The model under review builds one solid part; all positions refer to its coordinate system, in mm. Give positions to 0.01 mm unless a question says otherwise; leave off trailing zeros. Order: outer loops, then holes, each group sorted by start corner. A loop starts at its lowest first (then second) coordinate and runs counter-clockwise, first axis right, second up. Notation, with made-up numbers: (-33, -9.5) - (10, -9.5) arc R30 ccw to (10, 23.5) - close; hole circle Ø3 at (14.5, 25). An arc over 180 degrees is marked (long way). Put each result on its own line as item: value.
```python
from build123d import *

# Parameters (mm, degrees)
ESQUISSE4_R        = 1.55
ESQUISSE4_R_2      = 4
ESQUISSE4_R_3      = 5
ESQUISSE4_R_4      = 1.35255
ESQUISSE4_R_5      = 2.7051
BOSS_EXTRU_3_DEPTH = 3


with BuildPart() as part:
    # Esquisse4 → Boss.-Extru.3 (new body)
    with BuildSketch(Plane(origin=(0, 0, 0), x_dir=(0, 0, -1), z_dir=(1, 0, 0))):
        with BuildLine():
            Line((-40.60825, -12.7), (-40.60825, -16.144875))
            Line((-40.60825, -16.144875), (-40.60825, -16.348305132))
            add(Edge.make_bspline(
                [(-40.60825, -16.348305132), (-40.365634485, -16.661193605), (-40.112338127, -16.96547542), (-39.63020507, -17.593748723), (-39.400688032, -17.917191992), (-38.719045939, -18.893089111), (-38.271947044, -19.549593057), (-37.338540998, -20.831006808), (-36.855460104, -21.458516341), (-36.059725811, -22.342477591), (-35.781944124, -22.627029047), (-35.202868212, -23.17718548), (-34.900674383, -23.443503751), (-33.971943166, -24.212706181), (-33.324405882, -24.685383849), (-32.010805282, -25.604549776), (-31.348089528, -26.055770333), (-30.303090708, -26.660610546), (-29.948270215, -26.848696892), (-29.222483721, -27.184971005), (-28.851412004, -27.333773538), (-28.083597976, -27.570691368), (-27.685315555, -27.657976057), (-27.090666934, -27.715403346), (-26.891908645, -27.722631025), (-26.592836888, -27.712936491), (-26.492990431, -27.706278992), (-26.292963936, -27.685632014), (-26.192732932, -27.670522326), (-26.092449031, -27.65425)],
                knots=[0, 0, 0, 0, 0.0625, 0.0625, 0.125, 0.125, 0.25, 0.25, 0.375, 0.375, 0.4375, 0.4375, 0.5, 0.5, 0.625, 0.625, 0.75, 0.75, 0.8125, 0.8125, 0.875, 0.875, 0.9375, 0.9375, 0.96875, 0.96875, 0.984375, 0.984375, 1, 1, 1, 1], degree=3))
            Line((-26.092449031, -27.65425), (-26.092449031, -90))
            ThreePointArc((-26.092449031, -90), (2.64551669, -116.14013034), (25.954024412, -85.06135051))
            Line((25.954024412, -85.06135051), (25.954024412, -27.65425))
            add(Edge.make_bspline(
                [(25.954024412, -27.65425), (27.179118802, -27.419536533), (28.353377808, -27.051803075), (30.05705383, -26.34918771), (30.615126485, -26.089288473), (31.712904721, -25.521429223), (32.254485024, -25.212118815), (33.827204106, -24.230350536), (34.814025463, -23.502087852), (36.672007358, -21.907218093), (37.543320305, -21.040793316), (38.751902771, -19.623473398), (39.134714509, -19.134962989), (39.851014333, -18.131439591), (40.185535135, -17.615291382), (40.801362362, -16.550595558), (41.082635497, -16.002027673), (41.457015911, -15.150237789), (41.574249194, -14.86042264), (41.789713906, -14.277065554), (41.888049248, -13.98351322), (42.334688534, -12.506770959), (42.546239761, -11.296312151), (42.717568356, -9.451511475), (42.750611649, -8.83067761), (42.772859866, -7.900507946), (42.775360474, -7.590422151), (42.77555993, -6.970221998), (42.772087252, -6.66010067), (42.772087252, -6.35)],
                knots=[0, 0, 0, 0, 0.125, 0.125, 0.1875, 0.1875, 0.25, 0.25, 0.375, 0.375, 0.5, 0.5, 0.5625, 0.5625, 0.625, 0.625, 0.6875, 0.6875, 0.71875, 0.71875, 0.75, 0.75, 0.875, 0.875, 0.9375, 0.9375, 0.96875, 0.96875, 1, 1, 1, 1], degree=3))
            add(Edge.make_bspline(
                [(42.772087252, -6.35), (42.772087252, -5.874878454), (42.783792207, -5.398095979), (42.789657917, -4.447020546), (42.781867467, -3.973004463), (42.672546396, -2.563152451), (42.499179213, -1.637510108), (42.106282017, -0.267897459), (41.954068536, 0.185625042), (41.614819435, 1.087728793), (41.430081297, 1.530283034), (40.844911495, 2.839259084), (40.416604561, 3.689518781), (39.046783283, 6.190525131), (38.013123304, 7.787251584), (36.291657446, 10.082106977), (35.688509547, 10.830664164), (34.43654182, 12.281738953), (33.786199883, 12.985690235), (33.112075, 13.668565083)],
                knots=[0, 0, 0, 0, 0.0625, 0.0625, 0.125, 0.125, 0.25, 0.25, 0.3125, 0.3125, 0.375, 0.375, 0.5, 0.5, 0.75, 0.75, 0.875, 0.875, 1, 1, 1, 1], degree=3))
            add(Edge.make_bspline(
                [(33.112075, 13.668565083), (32.332207955, 14.539101946), (31.435060987, 15.277734234)],
                knots=[0, 0, 0, 1, 1, 1], degree=2))
            add(Edge.make_bspline(
                [(31.435060987, 15.277734234), (30.299691041, 16.309376592), (29.113704516, 17.275445235), (26.646604831, 19.084346085), (25.360475951, 19.928267183), (21.432297769, 22.265681686), (18.70167828, 23.563722979), (14.477833082, 25.213127628), (13.049229105, 25.71486416), (10.864398428, 26.369911185), (10.129061703, 26.571832136), (8.64156399, 26.936524394), (7.890831572, 27.098844789), (5.637990782, 27.512412208), (4.127431428, 27.693727696), (2.225306731, 27.768676851), (1.844136038, 27.775542931), (1.080940786, 27.779973661), (0.698904769, 27.777413484), (-0.446346689, 27.779064109), (-1.208874123, 27.797823926), (-2.732682239, 27.815308111), (-3.492085471, 27.806304753), (-5.004084105, 27.739990771), (-5.756994671, 27.684916502), (-8.006157922, 27.451797552), (-9.492662784, 27.204583891), (-11.701987236, 26.688775277), (-12.434852331, 26.491461598), (-13.894254142, 26.051929085), (-14.622118919, 25.807493497), (-16.765417144, 25.01223388), (-18.151500369, 24.400517874), (-20.847821735, 23.032525232), (-22.158708475, 22.277484827), (-24.716496252, 20.645447351), (-25.966430559, 19.7652326), (-28.39125747, 17.919703458), (-29.567431908, 16.954258357), (-31.287557173, 15.454109034), (-31.85380584, 14.945666112), (-32.972832423, 13.91291508), (-33.52577931, 13.388805977), (-34.066096443, 12.849822171)],
                knots=[0, 0, 0, 0, 0.0625, 0.0625, 0.125, 0.125, 0.25, 0.25, 0.3125, 0.3125, 0.34375, 0.34375, 0.375, 0.375, 0.4375, 0.4375, 0.453125, 0.453125, 0.46875, 0.46875, 0.5, 0.5, 0.53125, 0.53125, 0.5625, 0.5625, 0.625, 0.625, 0.65625, 0.65625, 0.6875, 0.6875, 0.75, 0.75, 0.8125, 0.8125, 0.875, 0.875, 0.9375, 0.9375, 0.96875, 0.96875, 1, 1, 1, 1], degree=3))
            add(Edge.make_bspline(
                [(-34.066096443, 12.849822171), (-35.159801618, 11.692162737), (-36.251081621, 10.53740284), (-37.166580532, 9.404947171)],
                knots=[0, 0, 0, 0, 1, 1, 1, 1], degree=3))
            ThreePointArc((-37.166580532, 9.404947171), (-37.363014685, 9.160281042), (-37.557796616, 8.914297524))
            add(Edge.make_bspline(
                [(-37.557796616, 8.914297524), (-38.142933539, 8.170182683), (-38.709522845, 7.412667282), (-39.741912272, 5.824816801), (-40.203133529, 4.998794666), (-40.60825, 4.142494902)],
                knots=[0, 0, 0, 0, 0.5, 0.5, 1, 1, 1, 1], degree=3))
            Line((-40.60825, 4.142494902), (-40.60825, -12.7))
        make_face()
        with Locations((0.1651, -103.128774516)):
            Circle(ESQUISSE4_R, mode=Mode.SUBTRACT)
        with Locations((-12.963674516, -90)):
            Circle(ESQUISSE4_R, mode=Mode.SUBTRACT)
        with Locations((0.1651, -90)):
            Circle(ESQUISSE4_R_2, mode=Mode.SUBTRACT)
        with Locations((-12.571436854, -77.1426291)):
            Circle(ESQUISSE4_R_3, mode=Mode.SUBTRACT)
        with Locations((0.1651, -76.871225484)):
            Circle(ESQUISSE4_R, mode=Mode.SUBTRACT)
        with Locations((13.293874516, -90)):
            Circle(ESQUISSE4_R, mode=Mode.SUBTRACT)
        with Locations((-16.9799, -14.9225)):
            Circle(ESQUISSE4_R_4, mode=Mode.SUBTRACT)
        with Locations((0.1651, -18.2245)):
            Circle(ESQUISSE4_R_5, mode=Mode.SUBTRACT)
        with BuildLine():
            Line((-6.1849, 11.646916554), (-6.1849, 6.103472306))
            ThreePointArc((-6.1849, 6.103472306), (0.1651, -0.246527694), (6.5151, 6.103472306))
            Line((6.5151, 6.103472306), (6.5151, 11.646916554))
            ThreePointArc((6.5151, 11.646916554), (16.056799278, 6.86795928), (22.793325, -1.408614826))
            Line((22.793325, -1.408614826), (23.12590424, -8.5725))
            Line((23.12590424, -8.5725), (17.3101, -8.5725))
            ThreePointArc((17.3101, -8.5725), (12.819971939, -10.432371939), (10.9601, -14.9225))
            Line((10.9601, -14.9225), (10.9601, -21.669375))
            Line((10.9601, -21.669375), (6.880225, -21.669375))
            Line((6.880225, -21.669375), (6.880225, -18.2245))
            ThreePointArc((6.880225, -18.2245), (0.1651, -11.509375), (-6.550025, -18.2245))
            Line((-6.550025, -18.2245), (-6.550025, -21.669375))
            Line((-6.550025, -21.669375), (-10.6299, -21.669375))
            Line((-10.6299, -21.669375), (-10.6299, -14.9225))
            ThreePointArc((-10.6299, -14.9225), (-12.489771939, -10.432371939), (-16.9799, -8.5725))
            Line((-16.9799, -8.5725), (-22.848998606, -8.5725))
            Line((-22.848998606, -8.5725), (-22.463125, -1.408614826))
            ThreePointArc((-22.463125, -1.408614826), (-15.726599278, 6.86795928), (-6.1849, 11.646916554))
        make_face(mode=Mode.SUBTRACT)
        with Locations((0.1651, 6.103472306)):
            Circle(ESQUISSE4_R_4, mode=Mode.SUBTRACT)
        with Locations((17.3101, -14.9225)):
            Circle(ESQUISSE4_R_4, mode=Mode.SUBTRACT)
    extrude(amount=BOSS_EXTRU_3_DEPTH)


solid = part.part
```
(1) Clearance check with flat-ended pins moving along their axes: pin 1 Ø1.5 at (x, y) = (1, 9.5) entering from -Z; pin 2 Ø0.9 at (x, y) = (2, -20) entering from +Z; pin 3 Ø0.9 at (x, z) = (2, 8) entering from +Y. State where each tip first meets the part, or that it passes through.
The answers:
pin 1: z = -37.28
pin 2: z = 38.26
pin 3: y = 27.48
(2) Wall thickness on L1, parallel to Y at x = 2.2, z = -2; L2, parallel to Z at x = 1.6, y = -91; L3, parallel to Z at x = 2.3, y = -29: over which ranges is each line inside the solid? List them lowest first.
The answers:
L1: -116.19 to -93.55, -86.45 to -20.21, -16.24 to -11.76, 0.02 to 27.77
L2: -26.4 to -14.48, -12.11 to -4.04, 3.71 to 11.78, 14.15 to 26.07
L3: -25.95 to 26.09
(3) Take a section at A-A, the plane y = -61.5. Write out the cut boundary in (x, z).
The answers:
outline: (0, -25.95) - (3, -25.95) - (3, 26.09) - (0, 26.09) - close
(4) Take a section at B-B, the plane x = 1.85. Count the separate pieces of the cut face and the enclosed holes in it, then the cut area to 3 significant figures.
The answers:
separate pieces: 1
enclosed holes: 11
area: 7,170 mm^2
